from build123d import *

# Parameters (mm, degrees)
SKETCH1_R                = 19
BOSS_EXTRUDE1_DEPTH      = 3.5
SKETCH2_R                = 30
SKETCH2_R_2              = 19
SKETCH2_R_3              = 2.8
BOSS_EXTRUDE2_DEPTH      = 11
BOSS_EXTRUDE3_DEPTH      = 2
BOSS_EXTRUDE3_DEPTH_BACK = 11
SKETCH4_R                = 2.9
SKETCH5_R                = 5
BOSS_EXTRUDE4_DEPTH      = 3
CUT_EXTRUDE1_START       = -10
SKETCH3_R                = 19
CUT_EXTRUDE1_DEPTH       = 10
CUT_EXTRUDE3_START       = -13
CUT_EXTRUDE3_DEPTH       = 13
FILLET1_R                = 10
FILLET2_R                = 5
CUT_EXTRUDE4_START       = -5
SKETCH8_R                = 4
SKETCH8_R_2              = 19
CUT_EXTRUDE4_DEPTH       = 11
FILLET3_R                = 1


with BuildPart() as part:
    # Sketch1 → Boss-Extrude1 (new body)
    with BuildSketch(Plane(origin=(0, 0, 0), x_dir=(1, 0, 0), z_dir=(0, 1, 0))):
        with Locations(Location((0, 0, 0), (0, 0, 270))):
            Circle(SKETCH1_R)
    extrude(amount=BOSS_EXTRUDE1_DEPTH)

    # Sketch2 → Boss-Extrude2 (add)
    with BuildSketch(Plane(origin=(0, 0, 0), x_dir=(1, 0, 0), z_dir=(0, 1, 0))):
        with Locations(Location((0, 0, 0), (0, 0, 270))):
            Circle(SKETCH2_R)
        with Locations(Location((0, 0, 0), (0, 0, 270))):
            Circle(SKETCH2_R_2, mode=Mode.SUBTRACT)
        with Locations(Location((0, 25, 0), (0, 0, 270))):
            Circle(SKETCH2_R_3, mode=Mode.SUBTRACT)
        with Locations(Location((21.650635095, -12.5, 0), (0, 0, 270))):
            Circle(SKETCH2_R_3, mode=Mode.SUBTRACT)
        with Locations(Location((-21.650635095, -12.5, 0), (0, 0, 270))):
            Circle(SKETCH2_R_3, mode=Mode.SUBTRACT)
    extrude(amount=BOSS_EXTRUDE2_DEPTH)

    # Sketch4 → Boss-Extrude3 (add, two sides: drawn at the far end of the back side and taken through both)
    with BuildSketch(Plane.XZ.offset(-BOSS_EXTRUDE3_DEPTH_BACK)):
        with Locations(Location((-21.650635095, 12.5, 0), (0, 0, 270))):
            Circle(SKETCH4_R)
        with Locations(Location((21.650635095, 12.5, 0), (0, 0, 270))):
            Circle(SKETCH4_R)
        with Locations(Location((0, -25, 0), (0, 0, 270))):
            Circle(SKETCH4_R)
    extrude(amount=BOSS_EXTRUDE3_DEPTH + BOSS_EXTRUDE3_DEPTH_BACK)

    # Sketch5 → Boss-Extrude4 (add)
    with BuildSketch(Plane(origin=(0, 11, 0), x_dir=(1, 0, 0), z_dir=(0, 1, 0))):
        with Locations((-26.103110985, -14.7860609)):
            Circle(SKETCH5_R)
        with Locations((0.246451131, 29.99898768)):
            Circle(SKETCH5_R)
        with Locations((25.856659853, -15.212926781)):
            Circle(SKETCH5_R)
    extrude(amount=-BOSS_EXTRUDE4_DEPTH)

    # Sketch3 → Cut-Extrude1 (cut)
    with BuildSketch(Plane(origin=(0, 3.5, 0), x_dir=(1, 0, 0), z_dir=(0, 1, 0)).offset(CUT_EXTRUDE1_START)):
        with Locations(Location((0, 0, 0), (0, 0, 270))):
            Circle(SKETCH3_R)
    extrude(amount=CUT_EXTRUDE1_DEPTH, mode=Mode.SUBTRACT)

    # Sketch7 → Cut-Extrude3 (cut)
    with BuildSketch(Plane(origin=(0, 11, 0), x_dir=(1, 0, 0), z_dir=(0, 1, 0)).offset(CUT_EXTRUDE3_START)):
        with BuildLine():
            ThreePointArc((-29.54423259, -5.20944533), (-25.980762114, 15), (-10.2606043, 28.190778624))
            Line((-10.2606043, 28.190778624), (-13.773984089, 37.84371026))
            Line((-13.773984089, 37.84371026), (-43.939319858, -7.747687605))
            Line((-43.939319858, -7.747687605), (-29.54423259, -5.20944533))
        make_face()
        with BuildLine():
            ThreePointArc((-26.13264562, -4.6078905), (-22.980662881, 13.267891901), (-9.075772579, 24.935480225))
            Line((-9.075772579, 24.935480225), (-10.2606043, 28.190778624))
            ThreePointArc((-10.2606043, 28.190778624), (-25.980762114, 15), (-29.54423259, -5.20944533))
            Line((-29.54423259, -5.20944533), (-26.13264562, -4.6078905))
        make_face()
        with BuildLine():
            Line((15.259965643, 41.926411025), (10.2606043, 28.190778624))
            ThreePointArc((10.2606043, 28.190778624), (25.980762114, 15), (29.54423259, -5.20944533))
            Line((29.54423259, -5.20944533), (39.660606503, -6.993234998))
            Line((39.660606503, -6.993234998), (15.259965643, 41.926411025))
        make_face()
        with BuildLine():
            Line((10.2606043, 28.190778624), (9.075772579, 24.935480225))
            ThreePointArc((9.075772579, 24.935480225), (21.736841548, 15.220300308), (26.535783801, 0))
            ThreePointArc((26.535783801, 0), (26.434807132, -2.312745947), (26.13264562, -4.6078905))
            Line((26.13264562, -4.6078905), (29.54423259, -5.20944533))
            ThreePointArc((29.54423259, -5.20944533), (25.980762114, 15), (10.2606043, 28.190778624))
        make_face()
        with BuildLine():
            Line((28.679354216, -34.17872342), (19.283628291, -22.981333294))
            ThreePointArc((19.283628291, -22.981333294), (0, -30), (-19.283628291, -22.981333294))
            Line((-19.283628291, -22.981333294), (-25.886622414, -30.850475262))
            Line((-25.886622414, -30.850475262), (28.679354216, -34.17872342))
        make_face()
        with BuildLine():
            Line((19.283628291, -22.981333294), (17.056873041, -20.327589725))
            ThreePointArc((17.056873041, -20.327589725), (0, -26.535783801), (-17.056873041, -20.327589725))
            Line((-17.056873041, -20.327589725), (-19.283628291, -22.981333294))
            ThreePointArc((-19.283628291, -22.981333294), (0, -30), (19.283628291, -22.981333294))
        make_face()
    extrude(amount=CUT_EXTRUDE3_DEPTH, mode=Mode.SUBTRACT)

    # Fillet1
    # the kernel refuses this fillet: 10 mm, written as the material it adds along each edge
    with BuildSketch(Plane(origin=(-26.13264562, 0, 4.6078905), x_dir=(-0.9848077530122318, 0, 0.17364817766679624), z_dir=(0, 1, 0)), Plane(origin=(17.056873041, 0, 20.327589725), x_dir=(0.6427876096865569, 0, 0.7660444431189634), z_dir=(0, 1, 0)), Plane(origin=(9.075772579, 0, -24.935480225), x_dir=(0.34202014332561265, 0, -0.9396926207859289), z_dir=(0, 1, 0))) as fillet1_piece_1:
        with BuildLine():
            CenterArc((9.045274498, -8.297697769), FILLET1_R, 123.92490422, 42.948020906)
            Line((-0.693413056, -6.026582466), (-0.888186807, -5.98116016))
            ThreePointArc((-0.888186807, -5.98116016), (-0.372612378, -3.01031053), (-0.2, 0))
            Line((-0.2, 0), (0, 0.2))
            ThreePointArc((0, 0.2), (1.732108099, 0.2), (3.352595033, 0.165953955))
            Line((3.352595033, 0.165953955), (3.464216199, 0))
        make_face()
    extrude(amount=11)
    with BuildSketch(Plane(origin=(-17.056873041, 0, 20.327589725), x_dir=(0.8344973728156843, 0, 0.551011918894429), z_dir=(0, 1, 0)), Plane(origin=(26.13264562, 0, 4.6078905), x_dir=(0.059941633142754296, 0, -0.99820188369697), z_dir=(0, 1, 0)), Plane(origin=(-9.075772579, 0, -24.935480225), x_dir=(-0.8944390059584274, 0, 0.44718996480254386), z_dir=(0, 1, 0))) as fillet1_piece_2:
        with BuildLine():
            CenterArc((7.20939257, -9.934457095), FILLET1_R, 96.563537437, 42.948020906)
            Line((-0.39597707, -3.441510719), (-0.548084463, -3.311651792))
            ThreePointArc((-0.548084463, -3.311651792), (-0.396677677, -1.697894369), (-0.198689142, 0.022860991))
            Line((-0.198689142, 0.022860991), (0.022860991, 0.198689142))
            ThreePointArc((0.022860991, 0.198689142), (3.03317152, 0.026076764), (6.04348205, 0.198689142))
            Line((6.04348205, 0.198689142), (6.06634304, 0))
        make_face()
    extrude(amount=11)

    # Fillet2
    fillet2_edges = [part.edges().sort_by_distance(p)[0] for p in [
        (-10.2606043, 5.5, -28.190778624),
        (-29.54423259, 5.5, 5.20944533),
        (-19.283628291, 5.5, 22.981333294),
        (19.283628291, 5.5, 22.981333294),
        (29.54423259, 5.5, 5.20944533),
        (10.2606043, 5.5, -28.190778624),
    ]]
    fillet(fillet2_edges, radius=FILLET2_R)

    # Sketch8 → Cut-Extrude4 (cut)
    with BuildSketch(Plane(origin=(0, 11, 0), x_dir=(1, 0, 0), z_dir=(0, 1, 0)).offset(CUT_EXTRUDE4_START)):
        with Locations((-16.524893724, 9.376987118)):
            Circle(SKETCH8_R)
        with Locations(Location((0, 0, 0), (0, 0, 42.512080704))):
            Circle(SKETCH8_R_2)
        with Locations((16.383155917, 9.622484201)):
            Circle(SKETCH8_R)
        with Locations((0.141737807, -18.999471319)):
            Circle(SKETCH8_R)
    extrude(amount=CUT_EXTRUDE4_DEPTH, mode=Mode.SUBTRACT)

    # Fillet3
    fillet3_edges = [part.edges().sort_by_distance(p)[0] for p in [
        (4.116263726, 8.5, 18.548756641),
        (-3.83907012, 8.5, 18.608104165),
        (14.005562597, 8.5, -12.839167276),
        (18.034625983, 8.5, -5.979319831),
        (-18.121826323, 8.5, -5.709589366),
        (-14.195555863, 8.5, -12.628784333),
    ]]
    fillet(fillet3_edges, radius=FILLET3_R)


solid = part.part
Can you work these out from the model? Positions are in its coordinate system, mm. A direction names the side the tool comes from. Give positions to 0.01 mm unless a question says otherwise; leave off trailing zeros. Loops run counter-clockwise (first coordinate to the right, second up) from the corner with the lowest first, then second, coordinate; pieces in that order, holes last. Notation, with made-up numbers: M -22.5,70.5 L -18.5,70.5 A25 ccw -18.5,105.5 Z; hole C 86,33 d11. An arc over 180 degrees is marked long. One line per item, written item: value. Start each with the question number.
1) I'm going to push flat-ended pins straight in: pin 1 (6 mm diameter, centred on y = 1.5, z = 8.5, fed in from -X); pin 2 (3.5 mm diameter, centred on x = 1, z = 20.5, fed in from +Y); pin 3 (3 mm diameter, centred on y = 3, z = 1, fed in from -X). Where does each tip first touch, or does it pass through?
2) If we section it at C-C, the plane z = -23.5: Write out the boundary of the cut face in (x, y).
3) If I drill on line 1 (Z direction, x = 0.5, y = 7.5); line 2 (Z direction, x = 0, y = 8.75); line 3 (X direction, y = 0.75, z = 4.5), over which ranges is the centre line in solid material (lowest first)? Write a range as [from, to].
4) Thinking about a two-plate mould opening in X: for faces 1 (the face through (22.89, 5.42, -13.42)), 2 (the face through (-30.51, 9.52, 17.15)), 3 (the face through (28, 8, 16)), which applies, +X half, -X half, draft (parallel to the pull), parting line (faces both ways), or undercut?
5) If we section it at D-D, the plane z = 12.5: Write out the boundary of the cut face in (x, y).
6) On a 3-axis mill with a long thin cutter (end or side, diameter ignored), from which of +Z, -Z, +X, -X, +Y, -Y can I reach the whole of each face in a straight line? I mean faces 4 (the face through (-23.42, -0.99, 14.8)), 5 (the face through (4, 11, -19)), 6 (the face through (-19.962, 8.465, -11.424)). Say none if no direction works.
7) If we section it at A-A, the plane z = 0: Write out the boundary of the cut face in (x, y).
8) If we section it at B-B, the plane x = 0: Write out the boundary of the cut face in (y, z), and give its area (3 significant figures).
Completed:
1. pin 1: stops at x = -29.13
1. pin 2: stops at y = 6
1. pin 3: stops at x = -27.55
2. outline: M -12.92,0 L -2.48,0 L -2.48,-2 L 2.48,-2 L 2.48,0 L 12.92,0 L 12.92,11 L -12.92,11 Z
3. line 1: z = [-30, -18.99], [22.98, 26.53]
3. line 2: z = [-34.99, -19], [23, 26.54]
3. line 3: x = [-28.71, -18.46], [18.46, 28.71]
4. face 1: +X half
4. face 2: undercut
4. face 3: draft
5. outline: M -30.55,8 L -27.27,8 L -27.27,0 L -24.55,0 L -24.55,-2 L -18.75,-2 L -18.75,0 L -14.31,0 L -14.31,11 L -30.55,11 Z; M 14.31,0 L 18.75,0 L 18.75,-2 L 24.55,-2 L 24.55,0 L 27.27,0 L 27.27,8 L 30.06,8 L 30.06,11 L 14.31,11 Z
6. face 4: -Y
6. face 5: +Z, -Z, +X, -X, +Y
6. face 6: +Y
7. outline: M -26.68,0 L -19,0 L -19,11 L -26.68,11 Z; M 19,0 L 26.68,0 L 26.68,11 L 19,11 Z
8. outline: M -2,-27.9 L 0,-27.9 L 0,-30 L 8,-30 L 8,-34.99 L 11,-34.99 L 11,-19 L 0,-19 L 0,-22.1 L -2,-22.1 Z; M 0,19 L 6,19 L 6,23 L 11,23 L 11,26.54 L 0,26.54 Z
8. area: 210 mm^2
